Work out the finished part from the listing and answer in its coordinate system (mm). A direction names the side the tool comes from. Coordinates: 2 decimals unless noted, no trailing zeros. Loops run counter-clockwise (first coordinate to the right, second up) from the corner with the lowest first, then second, coordinate; pieces in that order, holes last. Notation, with made-up numbers: (-31.5, -39) - (-26.5, -39) arc R21 ccw to (-26.5, -12) - close; hole circle Ø3 at (79.25, 76.25). An arc over 180 degrees is marked (long way). Write each question's results on one line, items separated by ' | '. Start each with the question number.
Item 1: Section B-B, the plane z = -24 is taken. Write down the section's boundary in (x, y).
Item 2: Section A-A, the plane y = 34 is taken. Write down the section's boundary in (x, z), plus the area to 3 significant figures.
Item 3: For a pull along Y with two mould halves and no side action, classify faces 6 (the face through (-56.85, 54.95, 14.3)), 7 (the face through (-5, 3, -16)), 8 (the face through (-40, 21, -34.5)) as +Y half, -Y half, draft (parallel to the pull), parting line (faces both ways), or undercut.
Item 4: Section C-C, the plane z = 15 is taken. Write down the section's boundary in (x, y), plus the area to 3 significant figures.
Item 5: Section D-D, the plane y = 23 is taken. Count the separate pieces of the cut face and the enclosed holes in it, plus the area to 3 significant figures.
Item 6: Consider probe 1 along X at (y, z) = (34, 9.25); probe 2 along Y at (x, z) = (-34, 15); probe 3 along X at (y, z) = (48, 23.5). Determine where each line is inside the solid, lowest interval first. Write a range as [from, to].
Item 7: A tool of negligible diameter and unlimited length cuts with its end or side. For faces 1 (the face through (-5, 21, -34.5)), 2 (the face through (-5, 43, -33)), 3 (the face through (-51.85, 12, -33)), 4 (the face through (-10.822, 12, -33)), 5 (the face through (-5, 23, -31.5)), from which of +Z, -Z, +X, -X, +Y, -Y can it reach the whole face along a straight path? Write none if from no direction.
Item 8: Each of these flat-tipped pins is pushed along its axis until it touches: pin 1 Ø10 at (x, z) = (-44, 21.5) entering from +Y; pin 2 Ø2.5 at (x, z) = (-3.5, -33.5) entering from +Y; pin 3 Ø11.5 at (x, z) = (-39, -18) entering from +Y. Where does it stop, or does it pass through?
from build123d import *

# Parameters (mm, degrees)
F0_R        = 31
F1_DEPTH    = 3
F2_W        = 22.7279674787
F2_H        = 3
F2_W_2      = 10.8224550456
F3_DEPTH    = 34.5
F4_W        = 10.8224550456
F4_H        = 3
F5_DEPTH    = 40
F6_W        = 22.7279674787
F6_H        = 3
F7_DEPTH    = 40
F8_DEPTH    = 27
F9_T1_DEPTH = 30
F10_SIZE    = 1


# Not quite as in the source:
# - a fillet or chamfer that OpenCascade refuses, or shapes differently, is made with other operations: its cross-section is extruded or revolved along the edge and cut away or added


with BuildPart() as f1:
    # F0 (on Top) → F1 (new body)
    with BuildSketch(Plane.XY):
        with BuildLine():
            ThreePointArc((-34, 0), (-9.9583694397, 9.9583694397), (0, 34))
            ThreePointArc((0, 34), (-50.5693336344, 63.6893446023), (-51.8504225243, 5.0627849352))
            ThreePointArc((-51.8504225243, 5.0627849352), (-43.2772487246, 1.2901749301), (-34, 0))
        make_face()
        with Locations((-34, 34)):
            Circle(F0_R, mode=Mode.SUBTRACT)
        with BuildLine():
            ThreePointArc((-34, 0), (-43.2772487246, 1.2901749301), (-51.8504225243, 5.0627849352))
            Line((-51.8504225243, 5.0627849352), (-51.8504225243, 0))
            Line((-51.8504225243, 0), (-34, 0))
        make_face()
        with BuildLine():
            Line((0, 0), (0, 34))
            ThreePointArc((0, 34), (-9.9583694397, 9.9583694397), (-34, 0))
            Line((-34, 0), (0, 0))
        make_face()
    extrude(amount=F1_DEPTH)

    # F2 (on face) → F3 (join)
    with BuildSketch(Plane(origin=(0, 0, 0), x_dir=(1, 0, 0), z_dir=(0, 0, -1))):
        with Locations((-40.4864387849, -1.5)):
            Rectangle(F2_W, F2_H)
        with Locations((-5.4112275228, -1.5)):
            Rectangle(F2_W_2, F2_H)
    extrude(amount=F3_DEPTH)

    # F4 (on face) → F5 (join)
    with BuildSketch(Plane(origin=(0, 3, 0), x_dir=(-1, 0, 0), z_dir=(0, 1, 0))):
        with Locations((5.4112275228, -33)):
            Rectangle(F4_W, F4_H)
    extrude(amount=F5_DEPTH)

    # F6 (on face) → F7 (join)
    with BuildSketch(Plane(origin=(0, 3, 0), x_dir=(-1, 0, 0), z_dir=(0, 1, 0))):
        with Locations((40.4864387849, -33)):
            Rectangle(F6_W, F6_H)
    extrude(amount=F7_DEPTH)

    # F8 (add): a face of the model
    f8_faces = [f1.faces().sort_by_distance(p)[0] for p in [
        (-50.1006821075, 62.8496031264, 3),
    ]]
    extrude(f8_faces, amount=F8_DEPTH)

    # F9: fillet of radius 10.3311475389 on 1 edges, made by hand

    # F9_s2 → F9_t1 (join)
    with BuildSketch(Plane.XY):
        with BuildLine():
            ThreePointArc((-55.6121599632, 7.7528184042), (-52.8843757474, 4.2873402421), (-51.8504225243, 0))
            Line((-51.8504225243, 0), (-51.8504225243, 5.0627849352))
            ThreePointArc((-51.8504225243, 5.0627849352), (-53.7770807796, 6.3437696741), (-55.6121599632, 7.7528184042))
        make_face()
    extrude(amount=F9_T1_DEPTH)

    # F10
    f10_edges = [f1.edges().sort_by_distance(p)[0] for p in [
        (-65, 34, 30),
    ]]
    chamfer(f10_edges, length=F10_SIZE)


solid = f1.part
Answer key:
1) outline: (-51.85, 0) - (-29.12, 0) - (-29.12, 3) - (-51.85, 3) - close; (-10.82, 0) - (0, 0) - (0, 3) - (-10.82, 3) - close
2) outline: (-68, 0) - (-65, 0) - (-65, 29) - (-66, 30) - (-68, 30) - close; (-51.85, -34.5) - (-29.12, -34.5) - (-29.12, -31.5) - (-51.85, -31.5) - close; (-10.82, -34.5) - (0, -34.5) - (0, -31.5) - (-10.82, -31.5) - close; (-3, 0) - (0, 0) - (0, 30) - (-2, 30) - (-3, 29) - close | area: 280 mm^2
3) face 6: undercut | face 7: +Y half | face 8: draft
4) outline: (-55.61, 7.75) arc R10.33 cw to (-51.85, 0) - (0, 0) - (0, 34) arc R34 ccw (long way) to start; hole circle Ø62 at (-34, 34) | area: 894 mm^2
5) separate pieces: 4 | enclosed holes: 0 | area: 346 mm^2
6) probe 1: x = [-68, -65], [-3, 0] | probe 2: y = [0, 3], [65, 68] | probe 3: x = [-64.98, -61.66], [-6.34, -3.02]
7) face 1: -Z, +X, -X, +Y, -Y | face 2: -Z, +X, -X, +Y | face 3: -Z, -X, +Y, -Y | face 4: -Z, +Y, -Y | face 5: +X, -X, +Y
8) pin 1: stops at y = 67.63 | pin 2: stops at y = 43 | pin 3: stops at y = 3
